Read the model definition and answer for the solid it produces. Units are mm, in the model's axes. Face numbers are marked on the shaded views. A direction names the side the tool comes from. Give positions to 0.01 mm unless a question says otherwise; leave off trailing zeros. Loops run counter-clockwise (first coordinate to the right, second up) from the corner with the lowest first, then second, coordinate; pieces in that order, holes last. Notation, with made-up numbers: (16.5, 48) -> (40.5, 48) arc R21 ccw to (40.5, 61) -> close; hole circle Ø1 at (32, 67). An arc over 180 degrees is marked (long way). Return JSON: item names as keys, results as strings. Group by question number.
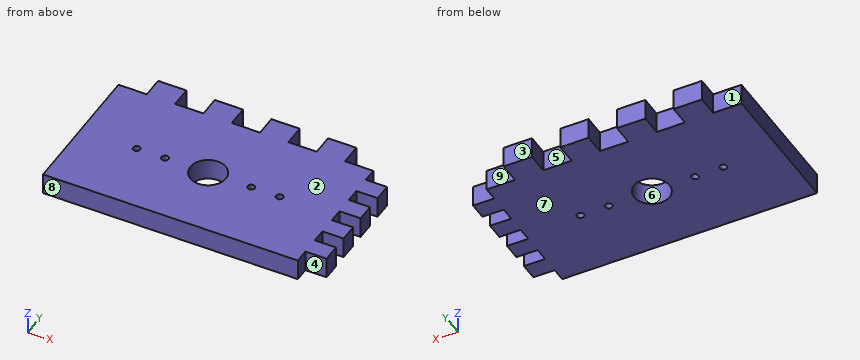
from build123d import *

# Parameters (mm, degrees)
SKETCH1_R           = 2.5
SKETCH1_R_2         = 0.5
BOSS_EXTRUDE1_DEPTH = 3


with BuildPart() as part:
    # Sketch1 → Boss-Extrude1 (new body)
    with BuildSketch(Plane.XY):
        Polygon((18, 10), (18, 8), (21, 8), (21, 5.5), (18, 5.5), (18, 3.5), (21, 3.5), (21, 1), (18, 1), (18, -1), (21, -1), (21, -3.5), (18, -3.5), (18, -5.5), (21, -5.5), (21, -8), (18, -8), (18, -10), (-18, -10), (-18, 10), (-14, 10), (-14, 13), (-10, 13), (-10, 10), (-6, 10), (-6, 13), (-2, 13), (-2, 10), (2, 10), (2, 13), (6, 13), (6, 10), (10, 10), (10, 13), (14, 13), (14, 10), align=None)
        Circle(SKETCH1_R, mode=Mode.SUBTRACT)
        with Locations((-6.09, 0)):
            Circle(SKETCH1_R_2, mode=Mode.SUBTRACT)
        with Locations((-10.09, 0)):
            Circle(SKETCH1_R_2, mode=Mode.SUBTRACT)
        with Locations(Location((10.09, 0, 0), (0, 0, 180))):
            Circle(SKETCH1_R_2, mode=Mode.SUBTRACT)
        with Locations(Location((6.09, 0, 0), (0, 0, 180))):
            Circle(SKETCH1_R_2, mode=Mode.SUBTRACT)
    extrude(amount=BOSS_EXTRUDE1_DEPTH)


solid = part.part
1. Flat-ended cylindrical pins translate along their axes: pin 1 Ø0.9 at (x, z) = (19.5, 1.5) entering from +Y; pin 2 Ø0.9 at (y, z) = (11.5, 1) entering from +X; pin 3 Ø0.9 at (x, z) = (8, 1) entering from +Y; pin 4 Ø4.5 at (x, y) = (0, 0) entering from -Z. Find the tip coordinate at first contact, or state that the pin passes through.
2. Which of the six approach directions +Z, -Z, +X, -X, +Y, -Y give full straight-line access (tool end or side, diameter ignored) to the marked faces 1, 2, 3, 4 and 5?
3. Section D-D on z = 2.6 is taken. State how many separate pieces and enclosed holes the cut face has, then the cut area to 3 significant figures.
4. Determine the mould class of the marked faces 6, 7, 8 and 9 for opening direction Y: pulls with the +Y half, pulls with the -Y half, needs draft (parallel to the pull), parting line crosses it, or undercut.
5. Section A-A on y = 0 is taken. Determine the outline of the cut face in (x, z).
6. Straight lines are drawn through the part: line 1 (Y direction, x = 0, z = 1.85); line 2 (Y direction, x = 10.09, z = 2.4); line 3 (X direction, y = -1.5, z = 1.7). For each, find the intervals that lie inside material, in ascending order. Write a range as from..to.
7. Section B-B on y = 11 is taken. Determine the outline of the cut face in (x, z), then the cut area to 3 significant figures.
8. Section C-C on x = 0 is taken. Determine the outline of the cut face in (y, z).
Completed:
{
 "1": {"pin 1": "stops at y = 8", "pin 2": "stops at x = 14", "pin 3": "stops at y = 10", "pin 4": "passes through"},
 "2": {"face 1": "+Z, -Z, -X, +Y", "face 2": "+Z, +X, -X, +Y, -Y", "face 3": "+Z, -Z, +X, -X, +Y", "face 4": "+Z, -Z, +X, -Y", "face 5": "+Z, -Z, +Y"},
 "3": {"separate pieces": "1", "enclosed holes": "5", "area": "775 mm²"},
 "4": {"face 6": "undercut", "face 7": "needs draft", "face 8": "pulls with the -Y half", "face 9": "pulls with the +Y half"},
 "5": {"outline": "(-18, 0) -> (-10.59, 0) -> (-10.59, 3) -> (-18, 3) -> close; (-9.59, 0) -> (-6.59, 0) -> (-6.59, 3) -> (-9.59, 3) -> close; (-5.59, 0) -> (-2.5, 0) -> (-2.5, 3) -> (-5.59, 3) -> close; (2.5, 0) -> (5.59, 0) -> (5.59, 3) -> (2.5, 3) -> close; (6.59, 0) -> (9.59, 0) -> (9.59, 3) -> (6.59, 3) -> close; (10.59, 0) -> (18, 0) -> (18, 3) -> (10.59, 3) -> close"},
 "6": {"line 1": "y = -10..-2.5, 2.5..10", "line 2": "y = -10..-0.5, 0.5..13", "line 3": "x = -18..-2, 2..21"},
 "7": {"outline": "(-14, 0) -> (-10, 0) -> (-10, 3) -> (-14, 3) -> close; (-6, 0) -> (-2, 0) -> (-2, 3) -> (-6, 3) -> close; (2, 0) -> (6, 0) -> (6, 3) -> (2, 3) -> close; (10, 0) -> (14, 0) -> (14, 3) -> (10, 3) -> close", "area": "48.0 mm²"},
 "8": {"outline": "(-10, 0) -> (-2.5, 0) -> (-2.5, 3) -> (-10, 3) -> close; (2.5, 0) -> (10, 0) -> (10, 3) -> (2.5, 3) -> close"}
}
